Autodesk Inventor part; units mm, degrees
ref_plane "YZ Plane" through (0, 0, 0) normal (1, 0, 0) x (0, 1, 0)
ref_plane "XZ Plane" through (0, 0, 0) normal (0, 1, 0) x (-1, 0, 0)
ref_plane "XY Plane" through (0, 0, 0) normal (0, 0, 1) x (1, 0, 0)
sketch "Sketch1" plane through (0, 0, 0) normal (0, 0, 1) x (1, 0, 0)
  arc A0 (7.3638, -36.4581) -> (12.7537, -40.2088) centre (11.3638, -36.4581) ccw
  arc A1 (12.7537, -40.2088) -> (35.5951, 21.83) centre (-2.3616, 0.5806) ccw
  arc A2 (35.5951, 21.83) -> (29.0406, 22.4471) centre (32.1048, 19.876) ccw
  line L0 (29.0406, 22.4471) -> (20.2358, 11.954)
  arc A3 (13.9161, 12.201) -> (20.2358, 11.954) centre (17.1717, 14.5251) ccw
  arc A4 (13.9161, 12.201) -> (6.2557, 18.6289) centre (-2.3616, 0.5806) ccw
  arc A5 (4.9149, 24.8097) -> (6.2557, 18.6289) centre (7.9791, 22.2386) ccw
  line L1 (4.9149, 24.8097) -> (13.7198, 35.3029)
  arc A6 (13.7198, 35.3029) -> (11.9738, 41.6506) centre (10.6556, 37.874) ccw
  arc A7 (11.9738, 41.6506) -> (-16.6971, 41.6506) centre (-2.3616, 0.5806) ccw
  arc A8 (-16.6971, 41.6506) -> (-18.443, 35.3029) centre (-15.3789, 37.874) ccw
  line L2 (-18.443, 35.3029) -> (-9.6382, 24.8097)
  arc A9 (-10.979, 18.6289) -> (-9.6382, 24.8097) centre (-12.7024, 22.2386) ccw
  arc A10 (-10.979, 18.6289) -> (-18.6394, 12.201) centre (-2.3616, 0.5806) ccw
  arc A11 (-24.9591, 11.954) -> (-18.6394, 12.201) centre (-21.8949, 14.5251) ccw
  line L3 (-24.9591, 11.954) -> (-33.7639, 22.4471)
  arc A12 (-33.7639, 22.4471) -> (-40.3184, 21.83) centre (-36.8281, 19.876) ccw
  arc A13 (-40.3184, 21.83) -> (-17.477, -40.2088) centre (-2.3616, 0.5806) ccw
  arc A14 (-17.477, -40.2088) -> (-12.0871, -36.4581) centre (-16.0871, -36.4581) ccw
  line L4 (-12.0871, -36.4581) -> (-12.0871, -12.1952)
  arc A15 (-6.4512, -8.5449) -> (-12.0871, -12.1952) centre (-8.0871, -12.1952) ccw
  arc A16 (-6.4512, -8.5449) -> (1.7279, -8.5449) centre (-2.3616, 0.5806) ccw
  arc A17 (7.3638, -12.1952) -> (1.7279, -8.5449) centre (3.3638, -12.1952) ccw
  line L5 (7.3638, -12.1952) -> (7.3638, -36.4581)
  circle A18 centre (-2.3616, 0.5806) radius 2.7
  circle A19 centre (29.9741, 13.9745) radius 2.6
  circle A20 centre (32.6384, 0.5806) radius 2.6
  circle A21 centre (29.9741, -12.8133) radius 2.6
  circle A22 centre (22.3871, -24.1682) radius 2.6
  circle A23 centre (11.0323, -31.7552) radius 2.6
  circle A24 centre (-34.6974, 13.9745) radius 2.6
  circle A25 centre (-37.3616, 0.5806) radius 2.6
  circle A26 centre (-34.6974, -12.8133) radius 2.6
  circle A27 centre (-27.1104, -24.1682) radius 2.6
  circle A28 centre (-15.7556, -31.7552) radius 2.6
  circle A29 centre (-2.3616, 35.5806) radius 2.6
  circle A30 centre (-2.3616, 0.5806) radius 38.1814
  point P0 (0, 0)
  point P1 (7.3638, -36.3414)
  point P2 (28.9846, 22.3804)
  point P3 (13.6637, 35.2361)
  point P4 (-18.387, 35.2361)
  point P5 (-33.7079, 22.3804)
  point P6 (-12.0871, -36.3414)
extrude "Extrusion1" add sketch "Sketch1" along normal blind 1.5 contours L5 A17 A16 A15 L4 A30 L3 A11 A10 A9 L2 L1 A5 A4 A3 L0 | A19 | A20 | A21 | A22 | A23 | A24 | A25 | A26 | A27 | A28 | A29
fillet "Fillet1" radius 4 6 edges at (13.6637, 35.2361, 0.75) (28.9846, 22.3804, 0.75) (7.3638, -36.3414, 0.75) (-12.0871, -36.3414, 0.75) (-18.387, 35.2361, 0.75) (-33.7079, 22.3804, 0.75)
sketch "Sketch2" plane through (0, 0, 0) normal (0, 0, -1) x (-1, 0, 0)
  circle A0 centre (2.3616, 0.5806) radius 2.7
  circle A1 centre (2.3616, 0.5806) radius 7.0777
  point P0 (0, 0)
extrude "Extrusion2" add sketch "Sketch2" along normal blind 6
properties part number "LED Diffuser_3DPrint"
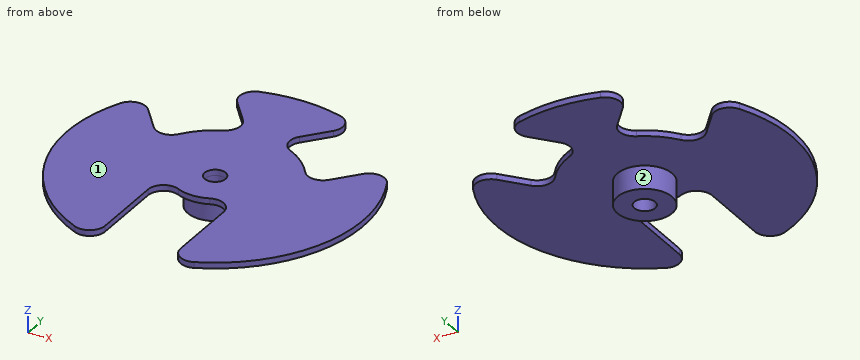
Build history of the part. All positions in model axes, mm. Face numbers are marked on the shaded views. A direction names the side the tool comes from. Round coordinates to 2 decimals unless told otherwise and drop trailing zeros. Write each loop counter-clockwise with the first axis right and the second up, starting at its lowest first coordinate (ties: lowest second). Pieces come first, ordered by that corner, then holes. Notation, with made-up numbers: (-37.5, -5) -> (-30.5, -5) arc R19 cw to (-30.5, 11) -> close; hole circle Ø8 at (80, -23.75). An arc over 180 degrees is marked (long way). Put each result on its own line as item: value.
Item 1: Tool access for the marked faces 1 and 2: list every direction of +Z, -Z, +X, -X, +Y, -Y with a clear straight run to the whole face (end or side of a thin tool).
Here are the results:
face 1: +Z, +X, -X, +Y, -Y
face 2: -Z
Item 2: Slice it at B-B, the plane x = -33.5. Give the cut face in (y, z).
Here are the results:
outline: (-21.52, 0) -> (19.45, 0) -> (19.45, 1.5) -> (-21.52, 1.5) -> close
Item 3: Flat gauge pins, fed straight in: P1, Ø10, axis at x = -32, y = -3, coming from the -Z side; P2, Ø2, axis at y = 0, z = -4, coming from the +X side; P3, Ø2, axis at x = 2, z = -4, coming from the -Y side; P4, Ø10, axis at x = 21, y = 25.5, coming from the +Z side. Where does each tip first touch, or does it go through?
Here are the results:
P1: stops at z = 0
P2: stops at x = 4.72
P3: stops at y = -5.65
P4: passes through
Item 4: Slice it at C-C, the plane z = -2.75. Give the cut face in (x, y), plus the area to 3 significant figures.
Here are the results:
outline: circle Ø14.16 at (-2.36, 0.58); hole circle Ø5.4 at (-2.36, 0.58)
area: 134 mm^2
Item 5: Wall check: probe 1 along Z at (x, y) = (30, -10); probe 2 along Y at (x, z) = (-0.5, 0.25); probe 3 along X at (y, z) = (-30.5, 0.75). Give the ranges that are in metal, low to high. Write a range as from..to.
Here are the results:
probe 1: z = 0..1.5
probe 2: y = -9.24..-1.38, 2.54..38.72
probe 3: x = -24.54..-12.09, 7.36..19.82
Item 6: Slice it at D-D, the plane y = 23.5. Give the cut face in (x, z), plus the area to 3 significant figures.
Here are the results:
outline: (-8.91, 0) -> (4.18, 0) -> (4.18, 1.5) -> (-8.91, 1.5) -> close
area: 19.6 mm^2
Item 7: Slice it at A-A, the plane y = -3.5. Give the cut face in (x, z).
Here are the results:
outline: (-40.32, 0) -> (-8.14, 0) -> (-8.14, -6) -> (3.42, -6) -> (3.42, 0) -> (35.6, 0) -> (35.6, 1.5) -> (-40.32, 1.5) -> close
